from build123d import *

# Parameters (mm, degrees)
F1_DEPTH = 4
F2_D     = 5
F3_R     = 3.5
F4_D     = 2.4
F5_SIZE  = 0.5
F6_R     = 5
F7_R     = 0.5


with BuildPart() as f1:
    # F0 (on Front) → F1 (new body)
    with BuildSketch(Plane.XZ):
        with BuildLine():
            Line((-36.3799407881, 6), (-40, -6))
            Line((-40, -6), (0, -6))
            Line((0, -6), (28, 0))
            Line((28, 0), (36, 0))
            ThreePointArc((36, 0), (39, 3), (36, 6))
            Line((36, 6), (-5, 6))
            Line((-5, 6), (-32, -1))
            Line((-32, -1), (-36.3799407881, 6))
        make_face()
    extrude(amount=-F1_DEPTH)

    # F2 (through all)
    with Locations(Plane.XZ):
        with Locations((0, 0)):
            Hole(F2_D / 2)

    # F3
    f3_edges = [f1.edges().sort_by_distance(p)[0] for p in [
        (-32, 2, -1),
    ]]
    fillet(f3_edges, radius=F3_R)

    # F4 (through all)
    with Locations(Plane.XZ):
        with Locations((36, 3)):
            Hole(F4_D / 2)

    # F5
    f5_edges = [f1.edges().sort_by_distance(p)[0] for p in [
        (-34.870592, 0, 3.587766),
        (-34.870592, 4, 3.587766),
    ]]
    chamfer(f5_edges, length=F5_SIZE)

    # F6
    f6_edges = [f1.edges().sort_by_distance(p)[0] for p in [
        (-40, 2, -6),
    ]]
    fillet(f6_edges, radius=F6_R)

    # F7
    f7_edges = [f1.edges().sort_by_distance(p)[0] for p in [
        (-36.379941, 2, 6),
    ]]
    fillet(f7_edges, radius=F7_R)


solid = f1.part
Verification items for the finished model (mm, model axes). A direction names the side the tool comes from. Coordinates: 2 decimals unless noted, no trailing zeros. Order: outer loops, then holes, each group sorted by start corner. A loop starts at its lowest first (then second) coordinate and runs counter-clockwise, first axis right, second up. Notation, with made-up numbers: M -0.75,68 L 16.25,68 A20 ccw 16.25,77 Z; hole C 54,63.25 d7. An arc over 180 degrees is marked long. Return JSON: item names as keys, results as strings.
1) Cross-section at D-D, the plane x = -15. Record the boundary of the cut face in (y, z).
Answer list:
{"outline": "M 0,-6 L 4,-6 L 4,2.89 L 3.5,3.41 L 0.5,3.41 L 0,2.89 Z"}
2) Cross-section at C-C, the plane z = -1.75. Record the boundary of the cut face in (x, y).
Answer list:
{"outline": "M -38.21,0 L -1.79,0 L -1.79,4 L -38.21,4 Z; M 1.79,0 L 19.83,0 L 19.83,4 L 1.79,4 Z"}
3) Access from +Z, -Z, +X, -X, +Y, -Y to the whole of each face (thin tool, end or side, straight path). Record for faces 1 (the flat face through (-34.907, 0.247, 3.168)), 2 (the flat face through (-37.368, 1.972, 2.726)), 3 (the flat face through (-16.08, 3.75, 2.87)), 4 (the flat face through (-34.56, 1.98, 3.09)).
Answer list:
{"face 1": "+Z, -Y", "face 2": "+Z, -X, +Y, -Y", "face 3": "+Z, +Y", "face 4": "+Z, +Y, -Y"}
4) Cross-section at B-B, the plane y = 2.85. Record the boundary of the cut face in (x, z), and give its area (3 significant figures).
Answer list:
{"outline": "M -38.06,0.44 A5 ccw -33.27,-6 L 0,-6 L 28,0 L 36,0 A3 ccw 36,6 L -5,6 L -29.52,-0.36 A3.5 cw -33.36,1.18 L -35.8,5.07 A0.5 ccw -36.7,4.95 Z; hole C 0,0 d5; hole C 36,3 d2.4", "area": "629 mm2"}
5) Cross-section at A-A, the plane x = -1.5. Record the boundary of the cut face in (y, z).
Answer list:
{"outline": "M 0,-6 L 4,-6 L 4,-2 L 0,-2 Z; M 0,2 L 4,2 L 4,6 L 0,6 Z"}
6) Release check for a two-part mould opening along Z. For faces 5 (the cylindrical face through (34.89, 2.03, 2.54)), 6 (the flat face through (32, 2, 0)), 7 (the cylindrical face through (-31.718, 2.021, -0.208)) record: +Z half, -Z half, draft (parallel to the pull), parting line (faces both ways), or undercut.
Answer list:
{"face 5": "undercut", "face 6": "-Z half", "face 7": "+Z half"}
7) Gauge pin test, flat end, axial feed: pin 1 (1 mm diameter, centred on x = 24, y = 3, fed in from -Z). Record the tip position at first contact, or that the pin passes through.
Answer list:
{"pin 1": "z = -0.96"}
8) Thickness scan on L1, parallel to Z at x = 0, y = 2.3; L2, parallel to Z at x = 36, y = 1; L3, parallel to Z at x = -29.5, y = 3.05. Record the ranges inside material, lowest first. Write a range as [from, to].
Answer list:
{"L1": "[-6, -2.5], [2.5, 6]", "L2": "[0, 1.8], [4.2, 6]", "L3": "[-6, -0.35]"}
